Geometry: final body of the model. Coordinates: model frame, mm. Face numbers are marked on the shaded views. A direction names the side the tool comes from. Coordinates: 2 decimals unless noted, no trailing zeros. Loops run counter-clockwise (first coordinate to the right, second up) from the corner with the lowest first, then second, coordinate; pieces in that order, holes last. Notation, with made-up numbers: (34, 10.25) - (69, 10.25) arc R32 cw to (69, 46.25) - close; hole circle Ø5 at (-20, 79). An arc over 180 degrees is marked (long way). Put each result on its own line as item: value. Start each with the question number.
1) Section B-B on x = -24.5. Output: boundary loops of the cut face in (y, z).
2) Material intervals for line 1 along X through (y, z) = (48.5, 51); line 2 along Z through (x, y) = (-67.5, -24.5), sorted ascending. Write a range as from..to.
3) Section C-C on z = 44. Output: boundary loops of the cut face in (x, y).
4) Section A-A on y = 0. Output: boundary loops of the cut face in (x, z), and give its area (3 significant figures).
5) Section D-D on x = 68.5. Output: boundary loops of the cut face in (y, z).
6) Contact query for flat-ended pins moving along their axis: pin 1 Ø3 at (y, z) = (31, 76.5) entering from -X; pin 2 Ø4 at (x, y) = (59.5, -21.5) entering from -Z; pin 3 Ø1 at (y, z) = (13.5, 1) entering from +X; pin 4 Ø4 at (x, y) = (61, 40) entering from +Z. Output: stop coordinate, or through.
7) Reachability of the marked faces 1 and 2 from +Z, -Z, +X, -X, +Y, -Y: full face, straight path, thin tool, end or side. Return the list, or none.
Autodesk Inventor part; units mm, degrees
ref_plane "YZ Plane" through (0, 0, 0) normal (1, 0, 0) x (0, 1, 0)
ref_plane "XZ Plane" through (0, 0, 0) normal (0, 1, 0) x (-1, 0, 0)
ref_plane "XY Plane" through (0, 0, 0) normal (0, 0, 1) x (1, 0, 0)
sketch "Sketch1" plane through (0, 0, 0) normal (0, 0, 1) x (1, 0, 0)
  line L0 (-77.5, -60) -> (77.5, -60)
  line L1 (77.5, -60) -> (77.5, 60)
  line L2 (77.5, 60) -> (-77.5, 60)
  line L3 (-77.5, 60) -> (-77.5, -60)
  line L4 (-77.5, -60) -> (77.5, 60) construction
  line L5 (77.5, -60) -> (-77.5, 60) construction
  point P0 (0, 0)
  dimension "d154" = 155
  dimension "d155" = 120
extrude "Plate3" add sketch "Sketch1" along normal blind 2
sketch "Sketch7" plane through (75.5, 60, 0) normal (1, 0, 0) x (0, 1, 0)
  line L0 (-120, 0) -> (0, 0)
  line L1 (0, 0) -> (0, 155)
  line L2 (0, 155) -> (-120, 155)
  line L3 (-120, 155) -> (-120, 0)
edge flange "Flange3" height 155 angle 90 thickness 2 bend radius 2.75 thickness toward (1, 0, 0) relief round relief width 2 relief depth 1 edges at (77.5, 0, 2) wall of the first edge with corners at (75.5, -60, 0) (75.5, 60, 0) (75.5, 60, 155) (75.5, -60, 155)
bend "Bend3"
corner "Corner3"
sketch "Sketch8" plane through (0, 0, 2) normal (0, 0, 1) x (1, 0, 0)
  line L0 (60, 50) -> (-60, 50)
  line L1 (-60, 50) -> (-60, -30)
  line L2 (-60, -30) -> (60, -30)
  line L3 (60, -30) -> (60, 50)
  line L4 (60, 50) -> (-60, -30) construction
  line L5 (-60, 50) -> (60, -30) construction
  line L6 (-77.5, 60) -> (72.75, 60)
  point P0 (0, 0)
  point P1 (0, 10)
  dimension "d166" = 120
  dimension "d167" = 80
  dimension "d168" = 10
extrude "Cut1" cut sketch "Sketch8" against normal blind 2
equation "\"БОРТ_стрингер_3_высота\" = 63"
equation "\"БОРТ_стрингер_4_высота\" = 48"
equation "\"БОРТ_стрингер_5_высота\" = 54"
equation "\"БОРТ_стрингер_6_высота\" = 81"
properties part number "MNT-CDF-503  main tube 1" material "Stainless Steel"
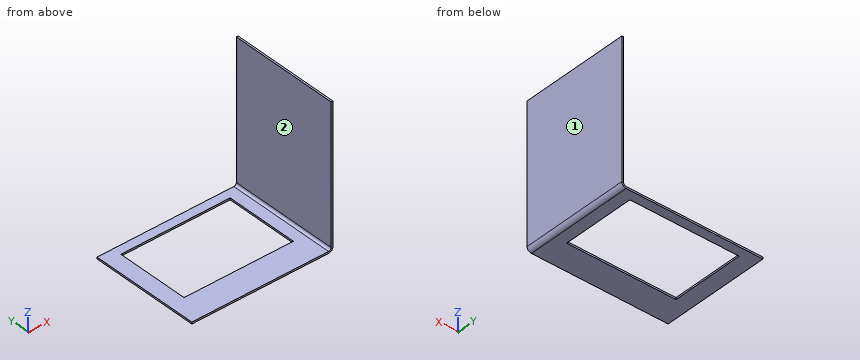
Answer block:
1. outline: (-60, 0) - (-30, 0) - (-30, 2) - (-60, 2) - close; (50, 0) - (60, 0) - (60, 2) - (50, 2) - close
2. line 1: x = 75.5..77.5
2. line 2: z = 0..2
3. outline: (75.5, -60) - (77.5, -60) - (77.5, 60) - (75.5, 60) - close
4. outline: (-77.5, 0) - (-60, 0) - (-60, 2) - (-77.5, 2) - close; (60, 0) - (72.75, 0) arc R4.75 ccw to (77.5, 4.75) - (77.5, 155) - (75.5, 155) - (75.5, 4.75) arc R2.75 cw to (72.75, 2) - (60, 2) - close
4. area: 373 mm²
5. outline: (-60, 0) - (60, 0) - (60, 2) - (-60, 2) - close
6. pin 1: stops at x = 75.5
6. pin 2: stops at z = 0
6. pin 3: stops at x = 76.21
6. pin 4: stops at z = 2
7. face 1: +Z, -Z, +X, +Y, -Y
7. face 2: +Z, -X, +Y, -Y
